Source: CAD feature listing. Evaluate the final solid. Frame: model axes, mm. Face numbers are marked on the shaded views. A direction names the side the tool comes from. Round coordinates to 2 decimals unless told otherwise and drop trailing zeros. Loops run counter-clockwise (first coordinate to the right, second up) from the corner with the lowest first, then second, coordinate; pieces in that order, holes last. Notation, with made-up numbers: (87.25, 26.5) -> (128.25, 26.5) arc R19 cw to (128.25, 33.5) -> close; hole circle Ø4 at (18, 44.5). An arc over 180 degrees is marked (long way). Put each result on its own line as item: value. Start each with the question number.
1. Material intervals for L1, parallel to X at y = -21, z = -15; L2, parallel to Z at x = 47.5, y = -16; L3, parallel to Y at x = -2.5, z = -5, sorted ascending.
2. Cut plane B-B (y = -4.5). Return the cut outline in (x, z), then the cut area to 3 significant figures.
3. Set-up query: the marked faces 5, 6 and 7. Return all of +Z, -Z, +X, -X, +Y, -Y with unobstructed straight access to the full face (end or side cutting, diameter ignored); none if empty.
4. Cut plane D-D (x = -7.5). Return the cut outline in (y, z), then the cut area to 3 significant figures.
5. Draft query along X for the marked faces 1, 2, 3 and 4. Return one class per face: pulls with the +X half, pulls with the -X half, needs draft (parallel to the pull), parting line crosses it, or undercut.
6. Cut plane A-A (y = -21.59). Return the cut outline in (x, z), then the cut area to 3 significant figures.
7. Contact query for flat-ended pins moving along their axis: pin 1 (4 mm diameter, centred on x = -9, z = -4, fed in from -Y); pin 2 (1.5 mm diameter, centred on y = -15.5, z = 1.5, fed in from -X); pin 3 (1 mm diameter, centred on y = -22, z = 10.5, fed in from -X); pin 4 (1 mm diameter, centred on x = -4.5, z = 4.5, fed in from -Y). Output: stop coordinate, or through.
8. Cut plane C-C (z = 10.5). Return the cut outline in (x, y), then the cut area to 3 significant figures.
```python
from build123d import *

# Parameters (mm, degrees)
F0_W     = 127
F0_H     = 25.4
F1_DEPTH = 2.54
F3_DEPTH = 38.1
F4_R     = 6.35
F5_DEPTH = 25.4


with BuildPart() as f1:
    # F0 (on Front) → F1 (new body)
    with BuildSketch(Plane.XZ):
        with Locations((-2.625061, -9.665867)):
            Rectangle(F0_W, F0_H)
    extrude(amount=F1_DEPTH)

    # F2 (on face) → F3 (join)
    with BuildSketch(Plane.XZ.offset(2.54)):
        with BuildLine():
            Line((-43.24917, -9.665867), (-66.125061, -9.665867))
            Line((-66.125061, -9.665867), (-66.125061, -22.365867))
            Line((-66.125061, -22.365867), (-2.625061, -22.365867))
            Line((-2.625061, -22.365867), (-2.625061, -9.665867))
            ThreePointArc((-2.625061, -9.665867), (-11.605317, -5.946123), (-15.325061, 3.034133))
            Line((-15.325061, 3.034133), (-21.675061, 3.034133))
            ThreePointArc((-21.675061, 3.034133), (-25.394805, -5.946123), (-34.375061, -9.665867))
            Line((-34.375061, -9.665867), (-43.24917, -9.665867))
        make_face()
        with BuildLine():
            ThreePointArc((16.424939, 3.034133), (-2.625061, 22.283079), (-21.675061, 3.034133))
            Line((-21.675061, 3.034133), (-15.325061, 3.034133))
            ThreePointArc((-15.325061, 3.034133), (-2.625061, 15.734133), (10.074939, 3.034133))
            Line((10.074939, 3.034133), (16.424939, 3.034133))
        make_face()
        with BuildLine():
            Line((-2.625061, -9.665867), (-2.625061, -22.365867))
            Line((-2.625061, -22.365867), (60.874939, -22.365867))
            Line((60.874939, -22.365867), (60.874939, -9.665867))
            Line((60.874939, -9.665867), (37.999048, -9.665867))
            Line((37.999048, -9.665867), (29.124939, -9.665867))
            ThreePointArc((29.124939, -9.665867), (20.144683, -5.946123), (16.424939, 3.034133))
            Line((16.424939, 3.034133), (10.074939, 3.034133))
            ThreePointArc((10.074939, 3.034133), (6.355195, -5.946123), (-2.625061, -9.665867))
        make_face()
    extrude(amount=F3_DEPTH)

    # F4 (on face) → F5 (cut)
    with BuildSketch(Plane.XY.offset(-9.665867)):
        with Locations((41.824939, -21.59)):
            Circle(F4_R)
        with Locations((-47.075061, -21.59)):
            Circle(F4_R)
    extrude(amount=-F5_DEPTH, mode=Mode.SUBTRACT)


solid = f1.part
```
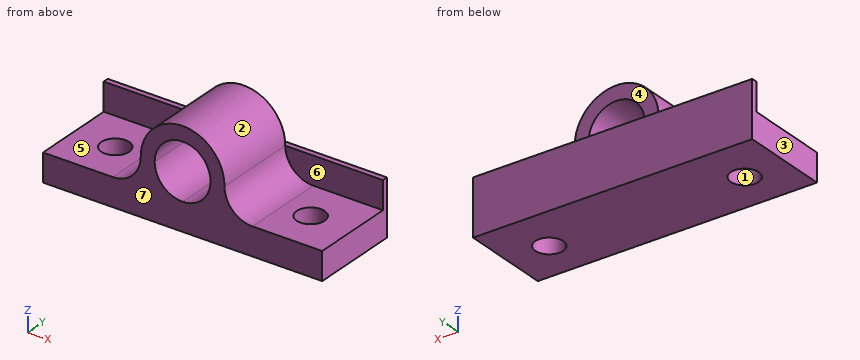
Solution:
1. L1: x = -66.13 to -53.4, -40.75 to 35.5, 48.15 to 60.87
1. L2: z = -22.37 to -9.67
1. L3: y = -2.54 to 0
2. outline: (-66.13, -22.37) -> (60.87, -22.37) -> (60.87, -9.67) -> (29.12, -9.67) arc R12.7 cw to (16.42, 3.03) arc R19.05 ccw (long way) to (-21.68, 3.03) arc R12.7 cw to (-34.38, -9.67) -> (-66.13, -9.67) -> close; hole circle Ø25.4 at (-2.63, 3.03)
2. area: 2,240 mm^2
3. face 5: +Z, -X, -Y
3. face 6: +Z, +X, -Y
3. face 7: +Z, -Z, +X, -X, -Y
4. outline: (-40.64, -22.37) -> (0, -22.37) -> (0, 3.03) -> (-2.54, 3.03) -> (-2.54, -8.69) -> (-40.64, -8.69) -> close; (-40.64, 14.76) -> (-2.54, 14.76) -> (-2.54, 21.65) -> (-40.64, 21.65) -> close
4. area: 848 mm^2
5. face 1: undercut
5. face 2: parting line crosses it
5. face 3: pulls with the -X half
5. face 4: needs draft
6. outline: (-66.13, -22.37) -> (-53.43, -22.37) -> (-53.43, -9.67) -> (-66.13, -9.67) -> close; (-40.73, -22.37) -> (35.47, -22.37) -> (35.47, -9.67) -> (29.12, -9.67) arc R12.7 cw to (16.42, 3.03) arc R19.05 ccw (long way) to (-21.68, 3.03) arc R12.7 cw to (-34.38, -9.67) -> (-40.73, -9.67) -> close; (48.17, -22.37) -> (60.87, -22.37) -> (60.87, -9.67) -> (48.17, -9.67) -> close; hole circle Ø25.4 at (-2.63, 3.03)
6. area: 1,910 mm^2
7. pin 1: stops at y = -2.54
7. pin 2: stops at x = -21.88
7. pin 3: stops at x = -20.43
7. pin 4: passes through
8. outline: (-20.24, -40.64) -> (-12.9, -40.64) -> (-12.9, -2.54) -> (-20.24, -2.54) -> close; (7.65, -40.64) -> (14.99, -40.64) -> (14.99, -2.54) -> (7.65, -2.54) -> close
8. area: 559 mm^2
